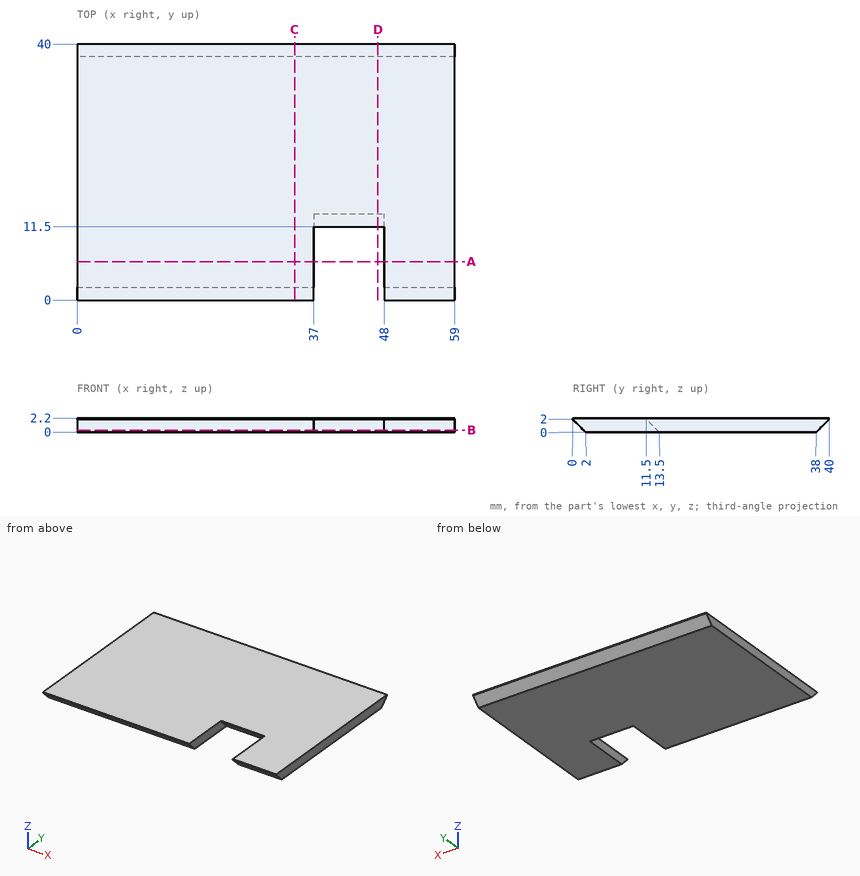
The drawing under review shows one solid part. Ordinate dimensions are in mm from its lowest x, y, z. Give positions to 0.01 mm unless a question says otherwise; leave off trailing zeros. Write each loop counter-clockwise with the first axis right and the second up, starting at its lowest first coordinate (ties: lowest second). Pieces come first, ordered by that corner, then holes.
1. Add section A-A, the plane y = 6. Write out the cut boundary in (x, z).
2. Add section C-C, the plane x = 34. Write out the cut boundary in (y, z).
3. Add section B-B, the plane z = 0.35. Write out the cut boundary in (x, y), plus the area to 3 significant figures.
4. Add section D-D, the plane x = 47. Write out the cut boundary in (y, z).
5. Wall thickness on L1, parallel to X at y = 7, z = 2; L2, parallel to Y at x = 30, z = 1.25; L3, parallel to Y at x = 42, z = 0.6: over which ranges is each line inside the solid? List them lowest first.
Worked answers:
1. outline: (0, 0) - (37, 0) - (37, 2.2) - (0, 2.2) - close; (48, 0) - (59, 0) - (59, 2.2) - (48, 2.2) - close
2. outline: (0, 2) - (2, 0) - (38, 0) - (40, 2) - (40, 2.2) - (0, 2.2) - close
3. outline: (0, 1.65) - (37, 1.65) - (37, 13.15) - (48, 13.15) - (48, 1.65) - (59, 1.65) - (59, 38.35) - (0, 38.35) - close
3. area: 2,040 mm2
4. outline: (11.5, 2) - (13.5, 0) - (38, 0) - (40, 2) - (40, 2.2) - (11.5, 2.2) - close
5. L1: x = 0 to 37, 48 to 59
5. L2: y = 0.75 to 39.25
5. L3: y = 12.9 to 38.6
